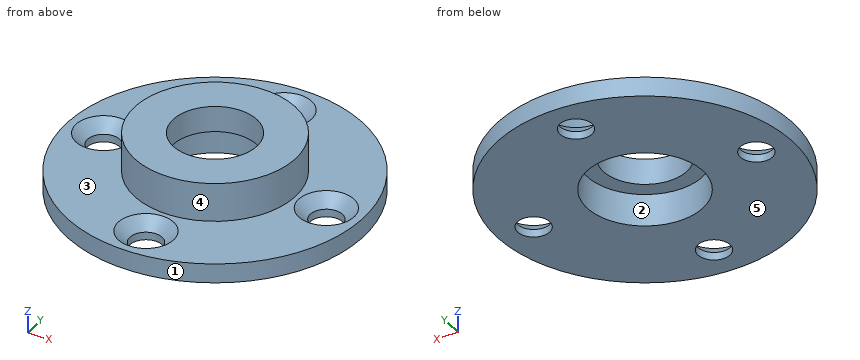
```python
from build123d import *

# Parameters (mm, degrees)
RIPETIZIONECIRCOLARE1_COUNT = 4


with BuildPart() as part:
    # Schizzo1 → Rivoluzione1 (revolve)
    with BuildSketch(Plane(origin=(0, 0, 0), x_dir=(1, 0, 0), z_dir=(0, 1, 0)), mode=Mode.PRIVATE) as rivoluzione1_sk:
        Polygon((6.5, 0), (6.5, 4), (9, 4), (9, 9), (23, 9), (23, 6), (12.5, 6), (12.5, 0), align=None)
    revolve(rivoluzione1_sk.sketch.rotate(Axis((0, 0, -7.574324324), (0, 0, 1)), 180), axis=Axis((0, 0, -7.574324324), (0, 0, 1)))

    # Schizzo4 → Foro svasato per Vite M6-2 (revolve, cut)
    with BuildSketch(Plane(origin=(0, 17.5, -6), x_dir=(0, -1, 0), z_dir=(1, 0, 0))):
        Polygon((0, 0), (0, 3), (2.5, 3), (2.5, 1.8), (4.3, 0), align=None)
    foro_svasato_per_vite_m6_2 = revolve(axis=Axis((0, 17.5, 0.35), (0, 0, -1)), mode=Mode.SUBTRACT)

    # RipetizioneCircolare1: Foro svasato per Vite M6-2 ×4 about axis
    ripetizionecircolare1_axis = Axis((0, 0, 0), (0, 0, 1))
    for i in range(1, RIPETIZIONECIRCOLARE1_COUNT):
        add(foro_svasato_per_vite_m6_2.rotate(ripetizionecircolare1_axis, i * 360 / RIPETIZIONECIRCOLARE1_COUNT), mode=Mode.SUBTRACT)


solid = part.part
```
Work out the finished part from the listing and answer in its coordinate system (mm). Face numbers are marked on the shaded views. A direction names the side the tool comes from. Round coordinates to 2 decimals unless told otherwise and drop trailing zeros. Write each loop counter-clockwise with the first axis right and the second up, starting at its lowest first coordinate (ties: lowest second). Pieces come first, ordered by that corner, then holes.
1) Determine the mould class of the marked faces 1, 2 and 3 for opening direction X: pulls with the +X half, pulls with the -X half, needs draft (parallel to the pull), parting line crosses it, or undercut.
2) A cutting plane is placed at D-D on x = -17.5. Determine the outline of the cut face in (y, z), and give its area (3 significant figures).
3) A cutting plane is placed at C-C on z = -7. Determine the outline of the cut face in (x, y), and give its area (3 significant figures).
4) Flat-ended cylindrical pins translate along their axes: P1, Ø1.5, axis at y = -2, z = -3.5, coming from the -X side; P2, Ø23, axis at x = 9, y = -5, coming from the +Z side; P3, Ø4, axis at x = 0, y = -17.5, coming from the +Z side; P4, Ø1.5, axis at x = 5, z = -6.5, coming from the +Y side. Find the tip coordinate at first contact, or state that the pin passes through.
5) A cutting plane is placed at A-A on x = 0. Determine the outline of the cut face in (y, z), and give its area (3 significant figures).
6) Which of the six approach directions +Z, -Z, +X, -X, +Y, -Y give full straight-line access (tool end or side, diameter ignored) to the marked faces 4 and 5?
7) Consider probe 1 along Z at (x, y) = (-5, 7); probe 2 along Z at (x, y) = (-17, -6.5); probe 3 along Y at (x, z) = (-0.5, -5.25). Determine where each line is inside the solid, lowest interval first.
Entries:
1. face 1: parting line crosses it
1. face 2: undercut
1. face 3: needs draft
2. outline: (-14.92, -9) - (-2.5, -9) - (-2.5, -7.8) - (-4.3, -6) - (-14.92, -6) - close; (2.5, -9) - (14.92, -9) - (14.92, -6) - (4.3, -6) - (2.5, -7.8) - close
2. area: 71.3 mm2
3. outline: circle Ø46 at (0, 0); hole circle Ø6.6 at (-17.5, 0); hole circle Ø18 at (0, 0); hole circle Ø6.6 at (0, -17.5); hole circle Ø6.6 at (0, 17.5); hole circle Ø6.6 at (17.5, 0)
3. area: 1,270 mm2
4. P1: stops at x = -12.44
4. P2: stops at z = 0
4. P3: passes through
4. P4: stops at y = 22.6
5. outline: (-23, -9) - (-20, -9) - (-20, -7.8) - (-21.8, -6) - (-23, -6) - close; (-15, -9) - (-9, -9) - (-9, -4) - (-6.5, -4) - (-6.5, 0) - (-12.5, 0) - (-12.5, -6) - (-13.2, -6) - (-15, -7.8) - close; (6.5, -4) - (9, -4) - (9, -9) - (15, -9) - (15, -7.8) - (13.2, -6) - (12.5, -6) - (12.5, 0) - (6.5, 0) - close; (20, -9) - (23, -9) - (23, -6) - (21.8, -6) - (20, -7.8) - close
5. area: 110 mm2
6. face 4: +Z
6. face 5: -Z, +X, -X, +Y, -Y
7. probe 1: z = -4 to 0
7. probe 2: z = -9 to -6
7. probe 3: y = -12.49 to -8.99, 8.99 to 12.49
